from build123d import *

# Parameters (mm, degrees)
BOSS_EXTRUDE1_DEPTH     = 18
CUT_EXTRUDE4_DEPTH      = 86.122527954
CUT_EXTRUDE4_DEPTH_BACK = 86.122527954
SKETCH7_R               = 4
SKETCH8_R               = 6.5
CUT_EXTRUDE5_DEPTH      = 18
CUT_EXTRUDE6_START      = -18
SKETCH10_R              = 6.5
CUT_EXTRUDE6_DEPTH      = 18
SKETCH12_R              = 4
CUT_EXTRUDE7_DEPTH      = 85.692648826


with BuildPart() as part:
    # Sketch1 → Boss-Extrude1 (new body)
    with BuildSketch(Plane.XY):
        with BuildLine():
            Line((0, -44.517412324), (0, -74.517412324))
            Line((0, -74.517412324), (-10, -74.517412324))
            Line((-10, -74.517412324), (-10, -44.517412324))
            add(Edge.make_bspline(
                [(-23.881707028, -26.938152673), (-18.294689626, -31.891258195), (-10, -36.821023575), (-10, -44.517412324)],
                knots=[0, 0, 0, 0, 1, 1, 1, 1], degree=3))
            ThreePointArc((-23.881707028, -26.938152673), (-35.855411942, 3.223264562), (-18.694362018, 30.765578635))
            ThreePointArc((-18.694362018, 30.765578635), (-11.589893335, 38.113065001), (-9, 48))
            Line((-9, 48), (-1, 48))
            Line((-1, 48), (-1, 27.982137159))
            ThreePointArc((-1, 27.982137159), (0, -28), (1, 27.982137159))
            Line((1, 27.982137159), (1, 48))
            Line((1, 48), (9, 48))
            ThreePointArc((9, 48), (11.589893335, 38.113065001), (18.694362018, 30.765578635))
            ThreePointArc((18.694362018, 30.765578635), (35.495463651, -6.006002016), (7.532125206, -35.203225561))
            ThreePointArc((7.532125206, -35.203225561), (2.11865956, -38.528109669), (0, -44.517412324))
        make_face()
    extrude(amount=BOSS_EXTRUDE1_DEPTH)

    # Sketch7 → Cut-Extrude4 (cut, two sides: drawn at the far end of the back side and taken through both)
    with BuildSketch(Plane.ZY.offset(-1).offset(-CUT_EXTRUDE4_DEPTH_BACK)):
        with Locations((9, 37.99106858)):
            Circle(SKETCH7_R)
    extrude(amount=CUT_EXTRUDE4_DEPTH + CUT_EXTRUDE4_DEPTH_BACK, mode=Mode.SUBTRACT)

    # Sketch8 → Cut-Extrude5 (cut)
    with BuildSketch(Plane(origin=(-9, 0, 0), x_dir=(0, 0, -1), z_dir=(1, 0, 0))):
        with Locations((-9, 37.99106858)):
            Circle(SKETCH8_R)
    extrude(amount=-CUT_EXTRUDE5_DEPTH, mode=Mode.SUBTRACT)

    # Sketch10 → Cut-Extrude6 (cut)
    with BuildSketch(Plane.ZY.offset(-9).offset(CUT_EXTRUDE6_START)):
        with Locations(Location((9, 37.99106858, 0), (0, 0, 180))):
            Circle(SKETCH10_R)
    extrude(amount=CUT_EXTRUDE6_DEPTH, mode=Mode.SUBTRACT)

    # Sketch12 → Cut-Extrude7 (cut, through all)
    with BuildSketch(Plane(origin=(0, 0, 0), x_dir=(0, 0, -1), z_dir=(1, 0, 0))):
        with Locations(Location((-9, -51.517412324, 0), (0, 0, 90))):
            Circle(SKETCH12_R)
        with Locations(Location((-9, -67.517412324, 0), (0, 0, 90))):
            Circle(SKETCH12_R)
    extrude(amount=-CUT_EXTRUDE7_DEPTH, mode=Mode.SUBTRACT)


solid = part.part
Geometry check sheet. Reference: the model listing, model coordinates, mm. A direction names the side the tool comes from. Coordinates: 2 decimals unless noted, no trailing zeros. Order: outer loops, then holes, each group sorted by start corner. A loop starts at its lowest first (then second) coordinate and runs counter-clockwise, first axis right, second up. Notation, with made-up numbers: (43.5, 19) - (66.5, 19) arc R30 ccw to (66.5, 55) - close; hole circle Ø8 at (70, 24). An arc over 180 degrees is marked (long way). Answer in a Markdown table with one row per item. Add a question column.
1) Release check for a two-part mould opening along Z. For faces 1 (the flat face through (1, 33, 9)), 2 (the cylindrical face through (-12.291, 31.646, 10.409)) record: +Z half, -Z half, draft (parallel to the pull), parting line (faces both ways), or undercut.
2) Gauge pin test, flat ends, axial feed: P1, Ø1, axis at y = -25, z = 5.5, coming from the +X side; P2, Ø6.5, axis at y = 37.99, z = 9, coming from the -X side; P3, Ø1.5, axis at y = 6.5, z = 16, coming from the +X side; P4, Ø5.5, axis at y = 40, z = 10.5, coming from the -X side. Record the tip position at first contact, or that the pin passes through.
3) Material ranges on line 1 along X through (y, z) = (0.5, 8.75); line 2 along Y through (x, z) = (-13.75, 9); line 3 along X through (y, z) = (-5.5, 6), recorded low to high. Write a range as [from, to].
4) Set-up check for faces 3 (the flat face through (-9, 41, 6)), 4 (the flat face through (9, 35, 6)), 5 (the flat face through (-10, -60, 9)), 6 (the flat face through (-1, 43, 9)), 7 (the flat face through (0, -59, 9)): record each of +Z, -Z, +X, -X, +Y, -Y from which the full face is reachable in a straight line by a thin tool's end or side.
5) Cross-section at A-A, the plane x = -7.5. Record the cut outline in (y, z), then the cut area to 3 significant figures.
6) Cross-section at C-C, the plane x = 20.5. Record the cut outline in (y, z), then the cut area to 3 significant figures.
7) Cross-section at D-D, the plane z = 6.75. State how many separate pieces and enclosed holes the cut face has, then the cut area to 3 significant figures.
8) Cross-section at B-B, the plane y = 11.5. Record the cut outline in (x, z), then the cut area to 3 significant figures.
Check result:
| question | item | result |
|---|---|---|
| 1 | face 1 | draft |
| 1 | face 2 | undercut |
| 2 | P1 | stops at x = 26.38 |
| 2 | P2 | passes through |
| 2 | P3 | stops at x = 35.54 |
| 2 | P4 | stops at x = -9 |
| 3 | line 1 | x = [-36, -28], [28, 36] |
| 3 | line 2 | y = [-35.87, -24.39], [24.39, 31.49] |
| 3 | line 3 | x = [-35.58, -27.45], [27.45, 35.58] |
| 4 | face 3 | -X |
| 4 | face 4 | +X |
| 4 | face 5 | +Z, -Z, -X, -Y |
| 4 | face 6 | +Z, -Z, +Y |
| 4 | face 7 | +Z, -Z, +X, -Y |
| 5 | outline | (-74.52, 0) - (-26.98, 0) - (-26.98, 18) - (-74.52, 18) - close; (26.98, 0) - (48, 0) - (48, 18) - (26.98, 18) - close; hole circle Ø8 at (-67.52, 9); hole circle Ø8 at (-51.52, 9); hole circle Ø8 at (37.99, 9) |
| 5 | area | 1,080 mm² |
| 6 | outline | (-29.59, 0) - (-19.07, 0) - (-19.07, 18) - (-29.59, 18) - close; (19.07, 0) - (29.59, 0) - (29.59, 18) - (19.07, 18) - close |
| 6 | area | 379 mm² |
| 7 | separate pieces | 5 |
| 7 | enclosed holes | 0 |
| 7 | area | 1,960 mm² |
| 8 | outline | (-34.11, 0) - (-25.53, 0) - (-25.53, 18) - (-34.11, 18) - close; (25.53, 0) - (34.11, 0) - (34.11, 18) - (25.53, 18) - close |
| 8 | area | 309 mm² |
